Autodesk Inventor part; units mm, degrees
ref_plane "YZ Plane" through (0, 0, 0) normal (1, 0, 0) x (0, 1, 0)
ref_plane "XZ Plane" through (0, 0, 0) normal (0, 1, 0) x (-1, 0, 0)
ref_plane "XY Plane" through (0, 0, 0) normal (0, 0, 1) x (1, 0, 0)
sketch "Sketch1" plane through (0, 0, 0) normal (0, 1, 0) x (-1, 0, 0)
  circle A0 centre (0, 0) radius 8
  dimension "d0" = 16
extrude "Extrusion1" add sketch "Sketch1" along normal blind 400
sketch "Sketch2" plane through (0, 0, 0) normal (0, -1, 0) x (1, 0, 0)
  circle A0 centre (0, 0) radius 8
extrude "Extrusion2" cut sketch "Sketch2" against normal blind 50
sketch "Sketch3" plane through (0, 50, 0) normal (0, -1, 0) x (1, 0, 0)
  circle A0 centre (0, 0) radius 8
extrude "Extrusion3" add sketch "Sketch3" along normal blind 50
sketch "Sketch4" plane through (0, 0, 0) normal (0, -1, 0) x (1, 0, 0)
  circle A0 centre (0, 0) radius 8
  circle A1 centre (0, 0) radius 6
  dimension "d7" = 12
extrude "Extrusion4" cut sketch "Sketch4" against normal blind 14
thread "Thread1"
sketch "Sketch6" plane through (0, 14, 0) normal (0, -1, 0) x (1, 0, 0)
  circle A0 centre (0, 0) radius 8
  circle A1 centre (0, 0) radius 6.05
  dimension "d13" = 12.1
extrude "Extrusion5" cut sketch "Sketch6" against normal blind 25
sketch "Sketch7" plane through (0, 0, 0) normal (0, -1, 0) x (1, 0, 0)
  circle A0 centre (0, 0) radius 6
  circle A1 centre (0, 0) radius 5
  dimension "d16" = 10
extrude "Extrusion6" add sketch "Sketch7" along normal blind 15 contours A1
sketch "Sketch8" plane through (0, 400, 0) normal (0, 1, 0) x (1, 0, 0)
  circle A0 centre (0, 0) radius 8
extrude "Extrusion7" cut sketch "Sketch8" against normal blind 27.101
sketch "Sketch9" plane through (0, 372.899, 0) normal (0, 1, 0) x (1, 0, 0)
  circle A0 centre (0, 0) radius 8
  circle A1 centre (0, 0) radius 5
  dimension "d21" = 10
extrude "Extrusion8" add sketch "Sketch9" along normal blind 12 contours A1
properties part number "1605_400mm"
For this review, take the finished solid that the model builds, in its own axes (mm). A direction names the side the tool comes from. Round coordinates to 2 decimals unless told otherwise and drop trailing zeros. Write each loop counter-clockwise with the first axis right and the second up, starting at its lowest first coordinate (ties: lowest second). Pieces come first, ordered by that corner, then holes. Notation, with made-up numbers: M -10,-5 L 4,-5 A16 cw 4,14 Z; hole C -19.75,2 d2. An arc over 180 degrees is marked long. Write item = value, one per line. Start each with the question number.
(1) For line 1 along Y through (x, z) = (-3.5, 6); line 2 along Z through (x, y) = (-0.75, 332); line 3 along X through (y, z) = (335, -4), list the stretches that pass through material, from the lowest coordinate up.
(2) Clearance check with flat-ended pins moving along their axes: pin 1 Ø3 at (y, z) = (162.5, 4.5) entering from +X; pin 2 Ø1.5 at (x, z) = (-5.5, 3) entering from -Y; pin 3 Ø2 at (x, z) = (-1, 6) entering from +Y. State where each tip first meets the part, or that it passes through.
(3) We need section C-C (y = 45.5). Give the boundary of the cut face in (x, z).
(4) We need section A-A (z = 0). Give the boundary of the cut face in (x, y), then the cut area to 3 significant figures.
(5) We need section B-B (x = 0). Give the boundary of the cut face in (y, z), then the cut area to 3 significant figures.
(6) For faces 1 (the face through (-0.1, 372.899, 5.2)), 2 (the face through (-1.08, -7.4, 4.88)), 3 (the face through (0, -15, 0)), list the 3-axis set-ups (+Z, -Z, +X, -X, +Y, -Y) from which the entire face can be reached by the end or side of a thin tool; tool diameter is ignored.
Results found:
q1.line_1 = 39 to 372.9
q1.line_2 = -7.96 to 7.96
q1.line_3 = -6.93 to 6.93
q2.pin_1 = 7.42
q2.pin_2 = 0
q2.pin_3 = 372.9
q3.outline = C 0,0 d16
q4.outline = M -8,39 L -6.05,39 L -6.05,14 L -6,14 L -6,0 L -5,0 L -5,-15 L 5,-15 L 5,0 L 6,0 L 6,14 L 6.05,14 L 6.05,39 L 8,39 L 8,372.9 L 5,372.9 L 5,384.9 L -5,384.9 L -5,372.9 L -8,372.9 Z
q4.area = 6,080 mm²
q5.outline = M -15,-5 L 0,-5 L 0,-6 L 14,-6 L 14,-6.05 L 39,-6.05 L 39,-8 L 372.9,-8 L 372.9,-5 L 384.9,-5 L 384.9,5 L 372.9,5 L 372.9,8 L 39,8 L 39,6.05 L 14,6.05 L 14,6 L 0,6 L 0,5 L -15,5 Z
q5.area = 6,080 mm²
q6.face_1 = +Y
q6.face_2 = -Y
q6.face_3 = +Z, -Z, +X, -X, -Y
